Work out the finished part from the listing and answer in its coordinate system (mm). A direction names the side the tool comes from. Round coordinates to 2 decimals unless told otherwise and drop trailing zeros. Loops run counter-clockwise (first coordinate to the right, second up) from the corner with the lowest first, then second, coordinate; pieces in that order, holes last.
```python
from build123d import *

# Parameters (mm, degrees)
SKETCH1_W           = 38
SKETCH1_H           = 41
BOSS_EXTRUDE1_DEPTH = 37
SKETCH2_W           = 30
SKETCH2_H           = 33
CUT_EXTRUDE1_DEPTH  = 14
SKETCH3_W           = 33
SKETCH3_H           = 20
CUT_EXTRUDE2_DEPTH  = 57.861674263
SKETCH4_W           = 9
SKETCH4_H           = 19
CUT_EXTRUDE3_DEPTH  = 37.197375595


with BuildPart() as part:
    # Sketch1 → Boss-Extrude1 (new body)
    with BuildSketch(Plane(origin=(0, 0, 0), x_dir=(1, 0, 0), z_dir=(0, 1, 0))):
        Rectangle(SKETCH1_W, SKETCH1_H)
    extrude(amount=BOSS_EXTRUDE1_DEPTH)

    # Sketch2 → Cut-Extrude1 (cut)
    with BuildSketch(Plane(origin=(0, 37, 0), x_dir=(1, 0, 0), z_dir=(0, 1, 0))):
        Rectangle(SKETCH2_W, SKETCH2_H)
    extrude(amount=-CUT_EXTRUDE1_DEPTH, mode=Mode.SUBTRACT)

    # Sketch3 → Cut-Extrude2 (cut, through all)
    with BuildSketch(Plane.ZY.offset(19)):
        with Locations((0, 10)):
            Rectangle(SKETCH3_W, SKETCH3_H)
    extrude(amount=-CUT_EXTRUDE2_DEPTH, mode=Mode.SUBTRACT)

    # Sketch4 → Cut-Extrude3 (cut, through all)
    with BuildSketch(Plane(origin=(0, 23, 0), x_dir=(1, 0, 0), z_dir=(0, 1, 0))):
        with Locations((-7.5, 0)):
            Rectangle(SKETCH4_W, SKETCH4_H)
    extrude(amount=-CUT_EXTRUDE3_DEPTH, mode=Mode.SUBTRACT)


solid = part.part
```
1. Find section B-B (z = 0). Write down the section's boundary in (x, y).
Answer key:
outline: (-19, 20) - (-12, 20) - (-12, 23) - (-15, 23) - (-15, 37) - (-19, 37) - close; (-3, 20) - (19, 20) - (19, 37) - (15, 37) - (15, 23) - (-3, 23) - close
2. Consider probe 1 along Z at (x, y) = (5.5, 15); probe 2 along X at (y, z) = (35, -7); probe 3 along X at (y, z) = (21, -8). Determine where each line is inside the solid, lowest interval first.
Answer key:
probe 1: z = -20.5 to -16.5, 16.5 to 20.5
probe 2: x = -19 to -15, 15 to 19
probe 3: x = -19 to -12, -3 to 19
3. Which of the six approach directions +Z, -Z, +X, -X, +Y, -Y give full straight-line access (tool end or side, diameter ignored) to faces 1 (the face through (15, 30, 0)), 2 (the face through (-8, 22, -9.5)), 3 (the face through (0, 10, -16.5))?
Answer key:
face 1: +Y
face 2: +Y, -Y
face 3: +X, -X, -Y
4. Determine the mould class of faces 4 (the face through (17, 37, 0)), 5 (the face through (0, 30, 16.5)), 6 (the face through (0, 18, -20.5)) for opening direction Z: +Z half, -Z half, draft (parallel to the pull), parting line (faces both ways), or undercut.
Answer key:
face 4: draft
face 5: undercut
face 6: -Z half
5. Find section C-C (y = 31). Write down the section's boundary in (x, z), then the cut area to 3 significant figures.
Answer key:
outline: (-19, -20.5) - (19, -20.5) - (19, 20.5) - (-19, 20.5) - close; hole (-15, -16.5) - (15, -16.5) - (15, 16.5) - (-15, 16.5) - close
area: 568 mm2
6. Find section A-A (y = 7). Write down the section's boundary in (x, z), then the cut area to 3 significant figures.
Answer key:
outline: (-19, -20.5) - (19, -20.5) - (19, -16.5) - (-19, -16.5) - close; (-19, 16.5) - (19, 16.5) - (19, 20.5) - (-19, 20.5) - close
area: 304 mm2
7. Given pin 1 (10 mm diameter, centred on x = 4, z = 2, fed in from -Y); pin 2 (4 mm diameter, centred on x = -5, z = -13, fed in from +Y), each flat-ended and moving along its own axis, determine where each tip first touches the part or whether it passes through.
Answer key:
pin 1: stops at y = 20
pin 2: stops at y = 23
8. Find section D-D (x = -14). Write down the section's boundary in (y, z).
Answer key:
outline: (0, -20.5) - (37, -20.5) - (37, -16.5) - (23, -16.5) - (23, 16.5) - (37, 16.5) - (37, 20.5) - (0, 20.5) - (0, 16.5) - (20, 16.5) - (20, -16.5) - (0, -16.5) - close
